```python
from build123d import *

# Parameters (mm, degrees)
SKETCH1_R           = 1.55
SKETCH1_R_2         = 1.6
BOSS_EXTRUDE1_DEPTH = 3
CUT_EXTRUDE3_REACH  = 131.236
SKETCH3_W           = 10
SKETCH3_H           = 6
BOSS_EXTRUDE2_DEPTH = 10
BOSS_EXTRUDE3_START = -206
SKETCH3_4_W         = 10
SKETCH3_4_H         = 6
BOSS_EXTRUDE3_DEPTH = 10
SKETCH3_6_R         = 2.1
CUT_EXTRUDE4_DEPTH  = 10
CUT_EXTRUDE5_START  = -196
SKETCH3_7_R         = 2.1
CUT_EXTRUDE5_DEPTH  = 10
CHAMFER1_SIZE       = 3


with BuildPart() as part:
    # Sketch1 → Boss-Extrude1 (new body)
    with BuildSketch(Plane(origin=(0, 0, 0), x_dir=(0, 1, 0), z_dir=(0, 0, 1))):
        with BuildLine():
            Line((-70, -103), (70, -103))
            ThreePointArc((70, -103), (75.656854249, -100.656854249), (78, -95))
            Line((78, -95), (78, 95))
            ThreePointArc((78, 95), (75.656854249, 100.656854249), (70, 103))
            Line((70, 103), (-70, 103))
            ThreePointArc((-70, 103), (-75.656854249, 100.656854249), (-78, 95))
            Line((-78, 95), (-78, -95))
            ThreePointArc((-78, -95), (-75.656854249, -100.656854249), (-70, -103))
        make_face()
        with Locations(Location((-68, -52.5, 0), (0, 0, 270))):
            Circle(SKETCH1_R, mode=Mode.SUBTRACT)
        with Locations(Location((-68, -85.5, 0), (0, 0, 270))):
            Circle(SKETCH1_R, mode=Mode.SUBTRACT)
        with Locations(Location((-10, -86.5, 0), (0, 0, 270))):
            Circle(SKETCH1_R, mode=Mode.SUBTRACT)
        with Locations(Location((-10, -56.5, 0), (0, 0, 270))):
            Circle(SKETCH1_R, mode=Mode.SUBTRACT)
        with Locations(Location((-68, -6.5, 0), (0, 0, 270))):
            Circle(SKETCH1_R, mode=Mode.SUBTRACT)
        with Locations(Location((-68, -39.5, 0), (0, 0, 270))):
            Circle(SKETCH1_R, mode=Mode.SUBTRACT)
        with Locations(Location((-10, -40.5, 0), (0, 0, 270))):
            Circle(SKETCH1_R, mode=Mode.SUBTRACT)
        with Locations(Location((-10, -10.5, 0), (0, 0, 270))):
            Circle(SKETCH1_R, mode=Mode.SUBTRACT)
        with Locations(Location((-68, 39.5, 0), (0, 0, 270))):
            Circle(SKETCH1_R, mode=Mode.SUBTRACT)
        with Locations(Location((-68, 6.5, 0), (0, 0, 270))):
            Circle(SKETCH1_R, mode=Mode.SUBTRACT)
        with Locations(Location((-10, 5.5, 0), (0, 0, 270))):
            Circle(SKETCH1_R, mode=Mode.SUBTRACT)
        with Locations(Location((-10, 35.5, 0), (0, 0, 270))):
            Circle(SKETCH1_R, mode=Mode.SUBTRACT)
        with Locations(Location((-68, 85.5, 0), (0, 0, 270))):
            Circle(SKETCH1_R, mode=Mode.SUBTRACT)
        with Locations(Location((-68, 52.5, 0), (0, 0, 270))):
            Circle(SKETCH1_R, mode=Mode.SUBTRACT)
        with Locations(Location((-10, 51.5, 0), (0, 0, 270))):
            Circle(SKETCH1_R, mode=Mode.SUBTRACT)
        with Locations(Location((-10, 81.5, 0), (0, 0, 270))):
            Circle(SKETCH1_R, mode=Mode.SUBTRACT)
        with Locations(Location((8.503950992, 0, 0), (0, 0, 270))):
            Circle(SKETCH1_R_2, mode=Mode.SUBTRACT)
        with Locations(Location((38.503950992, 20, 0), (0, 0, 270))):
            Circle(SKETCH1_R_2, mode=Mode.SUBTRACT)
        with Locations(Location((68.503950992, 0, 0), (0, 0, 270))):
            Circle(SKETCH1_R_2, mode=Mode.SUBTRACT)
        with Locations(Location((38.503950992, -20, 0), (0, 0, 270))):
            Circle(SKETCH1_R_2, mode=Mode.SUBTRACT)
    extrude(amount=BOSS_EXTRUDE1_DEPTH)

    # Sketch4 → Cut-Extrude3 (cut, up to next)
    with BuildSketch(Plane.XY.offset(3), mode=Mode.PRIVATE) as cut_extrude3_sk1:
        with BuildLine():
            Line((-78.5, -24), (-59.5, -24))
            ThreePointArc((-59.5, -24), (-57.378679656, -24.878679656), (-56.5, -27))
            Line((-56.5, -27), (-56.5, -51))
            ThreePointArc((-56.5, -51), (-57.378679656, -53.121320344), (-59.5, -54))
            Line((-59.5, -54), (-78.5, -54))
            ThreePointArc((-78.5, -54), (-80.621320344, -53.121320344), (-81.5, -51))
            Line((-81.5, -51), (-81.5, -27))
            ThreePointArc((-81.5, -27), (-80.621320344, -24.878679656), (-78.5, -24))
        make_face()
    cut_extrude3_tool1 = extrude(cut_extrude3_sk1.sketch, amount=-CUT_EXTRUDE3_REACH, mode=Mode.PRIVATE) & part.part
    # Sketch4 → Cut-Extrude3 (cut, up to next)
    with BuildSketch(Plane.XY.offset(3), mode=Mode.PRIVATE) as cut_extrude3_sk2:
        with BuildLine():
            Line((-35.5, -27), (-35.5, -51))
            ThreePointArc((-35.5, -51), (-34.621320344, -53.121320344), (-32.5, -54))
            Line((-32.5, -54), (-13.5, -54))
            ThreePointArc((-13.5, -54), (-11.378679656, -53.121320344), (-10.5, -51))
            Line((-10.5, -51), (-10.5, -27))
            ThreePointArc((-10.5, -27), (-11.378679656, -24.878679656), (-13.5, -24))
            Line((-13.5, -24), (-32.5, -24))
            ThreePointArc((-32.5, -24), (-34.621320344, -24.878679656), (-35.5, -27))
        make_face()
    cut_extrude3_tool2 = extrude(cut_extrude3_sk2.sketch, amount=-CUT_EXTRUDE3_REACH, mode=Mode.PRIVATE) & part.part
    # Sketch4 → Cut-Extrude3 (cut, up to next)
    with BuildSketch(Plane.XY.offset(3), mode=Mode.PRIVATE) as cut_extrude3_sk3:
        with BuildLine():
            Line((10.5, -27), (10.5, -51))
            ThreePointArc((10.5, -51), (11.378679656, -53.121320344), (13.5, -54))
            Line((13.5, -54), (32.5, -54))
            ThreePointArc((32.5, -54), (34.621320344, -53.121320344), (35.5, -51))
            Line((35.5, -51), (35.5, -27))
            ThreePointArc((35.5, -27), (34.621320344, -24.878679656), (32.5, -24))
            Line((32.5, -24), (13.5, -24))
            ThreePointArc((13.5, -24), (11.378679656, -24.878679656), (10.5, -27))
        make_face()
    cut_extrude3_tool3 = extrude(cut_extrude3_sk3.sketch, amount=-CUT_EXTRUDE3_REACH, mode=Mode.PRIVATE) & part.part
    # Sketch4 → Cut-Extrude3 (cut, up to next)
    with BuildSketch(Plane.XY.offset(3), mode=Mode.PRIVATE) as cut_extrude3_sk4:
        with BuildLine():
            Line((56.5, -27), (56.5, -51))
            ThreePointArc((56.5, -51), (57.378679656, -53.121320344), (59.5, -54))
            Line((59.5, -54), (78.5, -54))
            ThreePointArc((78.5, -54), (80.621320344, -53.121320344), (81.5, -51))
            Line((81.5, -51), (81.5, -27))
            ThreePointArc((81.5, -27), (80.621320344, -24.878679656), (78.5, -24))
            Line((78.5, -24), (59.5, -24))
            ThreePointArc((59.5, -24), (57.378679656, -24.878679656), (56.5, -27))
        make_face()
    cut_extrude3_tool4 = extrude(cut_extrude3_sk4.sketch, amount=-CUT_EXTRUDE3_REACH, mode=Mode.PRIVATE) & part.part
    # Sketch4 → Cut-Extrude3 (cut, up to next)
    with BuildSketch(Plane.XY.offset(3), mode=Mode.PRIVATE) as cut_extrude3_sk5:
        with BuildLine():
            Line((-7, 53.503950992), (7, 53.503950992))
            ThreePointArc((7, 53.503950992), (9.121320344, 52.625271335), (10, 50.503950992))
            Line((10, 50.503950992), (10, 26.503950992))
            ThreePointArc((10, 26.503950992), (9.121320344, 24.382630648), (7, 23.503950992))
            Line((7, 23.503950992), (-7, 23.503950992))
            ThreePointArc((-7, 23.503950992), (-9.121320344, 24.382630648), (-10, 26.503950992))
            Line((-10, 26.503950992), (-10, 50.503950992))
            ThreePointArc((-10, 50.503950992), (-9.121320344, 52.625271335), (-7, 53.503950992))
        make_face()
    cut_extrude3_tool5 = extrude(cut_extrude3_sk5.sketch, amount=-CUT_EXTRUDE3_REACH, mode=Mode.PRIVATE) & part.part
    add(cut_extrude3_tool1.solids().sort_by_distance((-69, -39, 3))[0], mode=Mode.SUBTRACT)
    add(cut_extrude3_tool2.solids().sort_by_distance((-23, -39, 3))[0], mode=Mode.SUBTRACT)
    add(cut_extrude3_tool3.solids().sort_by_distance((23, -39, 3))[0], mode=Mode.SUBTRACT)
    add(cut_extrude3_tool4.solids().sort_by_distance((69, -39, 3))[0], mode=Mode.SUBTRACT)
    add(cut_extrude3_tool5.solids().sort_by_distance((0, 38.503951, 3))[0], mode=Mode.SUBTRACT)

    # Sketch3 → Boss-Extrude2 (add)
    with BuildSketch(Plane.YZ.offset(103)):
        with Locations((-15.5, 3)):
            Rectangle(SKETCH3_W, SKETCH3_H)
        with Locations((15.5, 3)):
            Rectangle(SKETCH3_W, SKETCH3_H)
    extrude(amount=-BOSS_EXTRUDE2_DEPTH)

    # Sketch3<4> → Boss-Extrude3 (add)
    with BuildSketch(Plane.YZ.offset(103).offset(BOSS_EXTRUDE3_START)):
        with Locations((-15.5, 3)):
            Rectangle(SKETCH3_4_W, SKETCH3_4_H)
        with Locations((15.5, 3)):
            Rectangle(SKETCH3_4_W, SKETCH3_4_H)
    extrude(amount=BOSS_EXTRUDE3_DEPTH)

    # Sketch3<6> → Cut-Extrude4 (cut)
    with BuildSketch(Plane.YZ.offset(103)):
        with Locations(Location((-15.5, 3, 0), (0, 0, 270))):
            Circle(SKETCH3_6_R)
        with Locations(Location((15.5, 3, 0), (0, 0, 270))):
            Circle(SKETCH3_6_R)
    extrude(amount=-CUT_EXTRUDE4_DEPTH, mode=Mode.SUBTRACT)

    # Sketch3<7> → Cut-Extrude5 (cut)
    with BuildSketch(Plane.YZ.offset(103).offset(CUT_EXTRUDE5_START)):
        with Locations(Location((-15.5, 3, 0), (0, 0, 270))):
            Circle(SKETCH3_7_R)
        with Locations(Location((15.5, 3, 0), (0, 0, 270))):
            Circle(SKETCH3_7_R)
    extrude(amount=-CUT_EXTRUDE5_DEPTH, mode=Mode.SUBTRACT)

    # Chamfer1
    # the kernel refuses this chamfer: 3 mm, written as the material it adds along each edge
    with BuildSketch(Plane(origin=(93, -9.884951036, 3), x_dir=(-0.9996219169112968, 0, -0.027495876610586334), z_dir=(0, -1, 0))) as chamfer1_piece_1_section:
        Polygon((CHAMFER1_SIZE * 0.999621916911, -CHAMFER1_SIZE * 0.0274958766106), (-CHAMFER1_SIZE * 0.0274958766106, -CHAMFER1_SIZE * 0.999621916911), (0, 0), align=None)
    chamfer1_piece_1 = extrude(amount=10.615048964, mode=Mode.PRIVATE)
    chamfer1_piece_1 = split(chamfer1_piece_1, bisect_by=Plane(origin=(90.522066824, -10.5, 3.477933176), z_dir=(0, -1, 0)), keep=Keep.TOP, mode=Mode.PRIVATE)
    chamfer1_piece_1 = chamfer1_piece_1 - Plane(origin=(90.522066824, -15.5, 3), x_dir=(0, 0, -1), z_dir=(1, 0, 0)) * Cylinder(2.1, 34, mode=Mode.PRIVATE)
    add(chamfer1_piece_1)
    with BuildSketch(Plane(origin=(93, 21.115048964, 3), x_dir=(-0.9996219169112968, 0, -0.027495876610586334), z_dir=(0, -1, 0))) as chamfer1_piece_2_section:
        Polygon((CHAMFER1_SIZE * 0.999621916911, -CHAMFER1_SIZE * 0.0274958766106), (-CHAMFER1_SIZE * 0.0274958766106, -CHAMFER1_SIZE * 0.999621916911), (0, 0), align=None)
    chamfer1_piece_2 = extrude(amount=10.615048964, mode=Mode.PRIVATE)
    chamfer1_piece_2 = split(chamfer1_piece_2, bisect_by=Plane(origin=(90.522066824, 20.5, 3.477933176), z_dir=(0, -1, 0)), keep=Keep.TOP, mode=Mode.PRIVATE)
    chamfer1_piece_2 = chamfer1_piece_2 - Plane(origin=(90.522066824, 15.5, 3), x_dir=(0, 0, -1), z_dir=(1, 0, 0)) * Cylinder(2.1, 34, mode=Mode.PRIVATE)
    add(chamfer1_piece_2)
    with BuildSketch(Plane(origin=(-93, -9.884951036, 3), x_dir=(0.9996219169112968, 0, -0.027495876610586334), z_dir=(0, -1, 0))) as chamfer1_piece_3_section:
        Polygon((CHAMFER1_SIZE * 0.999621916911, CHAMFER1_SIZE * 0.0274958766106), (-CHAMFER1_SIZE * 0.0274958766106, CHAMFER1_SIZE * 0.999621916911), (0, 0), align=None)
    chamfer1_piece_3 = extrude(amount=10.615048964, mode=Mode.PRIVATE)
    chamfer1_piece_3 = split(chamfer1_piece_3, bisect_by=Plane(origin=(-90.522066824, -10.5, 3.477933176), z_dir=(0, -1, 0)), keep=Keep.TOP, mode=Mode.PRIVATE)
    chamfer1_piece_3 = chamfer1_piece_3 - Plane(origin=(-90.522066824, -15.5, 3), x_dir=(0, 0, -1), z_dir=(1, 0, 0)) * Cylinder(2.1, 34, mode=Mode.PRIVATE)
    add(chamfer1_piece_3)
    with BuildSketch(Plane(origin=(-93, 21.115048964, 3), x_dir=(0.9996219169112968, 0, -0.027495876610586334), z_dir=(0, -1, 0))) as chamfer1_piece_4_section:
        Polygon((CHAMFER1_SIZE * 0.999621916911, CHAMFER1_SIZE * 0.0274958766106), (-CHAMFER1_SIZE * 0.0274958766106, CHAMFER1_SIZE * 0.999621916911), (0, 0), align=None)
    chamfer1_piece_4 = extrude(amount=10.615048964, mode=Mode.PRIVATE)
    chamfer1_piece_4 = split(chamfer1_piece_4, bisect_by=Plane(origin=(-90.522066824, 20.5, 3.477933176), z_dir=(0, -1, 0)), keep=Keep.TOP, mode=Mode.PRIVATE)
    chamfer1_piece_4 = chamfer1_piece_4 - Plane(origin=(-90.522066824, 15.5, 3), x_dir=(0, 0, -1), z_dir=(1, 0, 0)) * Cylinder(2.1, 34, mode=Mode.PRIVATE)
    add(chamfer1_piece_4)


solid = part.part
```
Can you work these out from the model? Positions are in its coordinate system, mm. A direction names the side the tool comes from. Round coordinates to 2 decimals unless told otherwise and drop trailing zeros. Loops run counter-clockwise (first coordinate to the right, second up) from the corner with the lowest first, then second, coordinate; pieces in that order, holes last. Notation, with made-up numbers: (78.25, 54) -> (127.25, 54) arc R9 cw to (127.25, 66) -> close; hole circle Ø7 at (61, 63.25). An arc over 180 degrees is marked (long way). Answer in a Markdown table with one row per item.
Item 1: On a 3-axis mill with a long thin cutter (end or side, diameter ignored), from which of +Z, -Z, +X, -X, +Y, -Y can I reach the whole of each face in a straight line? I mean faces 4 (the flat face through (98, -16, 6)), 5 (the cylindrical face through (-97.85, 15.59, 5.1)), 6 (the cylindrical face through (98.04, -15.41, 5.1)). Say none if no direction works.
Answer block:
| item | result |
|---|---|
| face 4 | +Z, +X, -X, +Y, -Y |
| face 5 | -X |
| face 6 | +X |
Item 2: Suppose I cut it at B-B, the plane x = -45. List the corners of the cut face in (y, z) for me.
Answer block:
| item | result |
|---|---|
| outline | (-78, 0) -> (78, 0) -> (78, 3) -> (-78, 3) -> close |
Item 3: We'd pull the mould along Y, two halves only. Please class faces 1 (the cylindrical face through (100.594, -75.719, 1.479)), 2 (the flat face through (103, -1, 2)), 3 (the cylindrical face through (-97.85, -15.41, 5.1)): released by +Y, released by -Y, zero draft, split by the parting line, or undercut.
Answer block:
| item | result |
|---|---|
| face 1 | released by -Y |
| face 2 | zero draft |
| face 3 | undercut |
Item 4: Will these pins go through, and if not, where does the flat tip stop? P1, Ø12, axis at x = -30.5, y = 23.5, coming from the +Z side; P2, Ø0.9, axis at x = 97, z = 5, coming from the -Y side; P3, Ø1.5, axis at x = -98, z = 4, coming from the +Y side.
Answer block:
| item | result |
|---|---|
| P1 | z = 3 |
| P2 | y = -20.5 |
| P3 | y = 20.5 |
Item 5: If I drill on probe 1 along Y at (x, z) = (6.5, 0.7); probe 2 along X at (y, z) = (-42, 0.7); probe 3 along Y at (x, z) = (29, 2.75), over which ranges is the centre line in solid material (lowest first)?
Answer block:
| item | result |
|---|---|
| probe 1 | -78 to -69.55, -66.45 to 23.5, 53.5 to 78 |
| probe 2 | -103 to -81.5, -56.5 to -35.5, -10.5 to 10.5, 35.5 to 56.5, 81.5 to 103 |
| probe 3 | -78 to -54, -24 to 78 |
Item 6: Suppose I cut it at A-A, the plane y = 15.5. List the corners of the cut face in (x, z) for me.
Answer block:
| item | result |
|---|---|
| outline | (-103, 0) -> (103, 0) -> (103, 0.9) -> (93, 0.9) -> (93, 3) -> (-93, 3) -> (-93, 0.9) -> (-103, 0.9) -> close; (-103, 5.1) -> (-92.1, 5.1) -> (-93, 6) -> (-103, 6) -> close; (92.1, 5.1) -> (103, 5.1) -> (103, 6) -> (93, 6) -> close |
